Input: part model. Units: mm. Frame: model coordinates. A direction names the side the tool comes from. Coordinates: 2 decimals unless noted, no trailing zeros. Write each loop counter-clockwise with the first axis right and the second up, starting at its lowest first coordinate (ties: lowest second). Pieces come first, ordered by that corner, then holes. Notation, with made-up numbers: (-24.5, -28.75) - (-3.5, -28.75) arc R21 ccw to (-3.5, -22.75) - close; hole circle Ø6 at (66, 74). An arc over 180 degrees is marked (long way). Use CSV: the item, a comma, the result in double quotes.
```python
from build123d import *

# Parameters (mm, degrees)
BOSS_EXTRUDE1_DEPTH                             = 7.62
SKETCH11_W                                      = 17.78
SKETCH11_H                                      = 17.78
CUT_EXTRUDE1_DEPTH                              = 3.175
SKETCH12_W                                      = 3.81
SKETCH12_H                                      = 60.325
CUT_EXTRUDE2_DEPTH                              = 96.139869666
SKETCH14_W                                      = 7.62
SKETCH14_H                                      = 8.255
BOSS_EXTRUDE3_DEPTH                             = 3.175
SKETCH24_W                                      = 7.62
SKETCH24_H                                      = 6.35
BOSS_EXTRUDE4_DEPTH                             = 1.27
CSK_FOR_M3_FLAT_HEAD_MACHINE_SCREW2_D           = 3.4
CSK_FOR_M3_FLAT_HEAD_MACHINE_SCREW2_CSINK_D     = 6.3
CSK_FOR_M3_FLAT_HEAD_MACHINE_SCREW2_CSINK_ANGLE = 90
CSK_FOR_M3_FLAT_HEAD_MACHINE_SCREW3_D           = 3.4
CSK_FOR_M3_FLAT_HEAD_MACHINE_SCREW3_CSINK_D     = 6.3
CSK_FOR_M3_FLAT_HEAD_MACHINE_SCREW3_CSINK_ANGLE = 90
F_4_40_TAPPED_HOLE2_D                           = 2.2606
F_4_40_TAPPED_HOLE2_DEPTH                       = 8.8646
F_4_40_TAPPED_HOLE2_TIP                         = 0.679152758
SKETCH25_W                                      = 5.08
SKETCH25_H                                      = 93.98
CUT_EXTRUDE3_DEPTH                              = 96.139869666
FILLET1_R                                       = 3.302


with BuildPart() as part:
    # Sketch1 → Boss-Extrude1 (new body)
    with BuildSketch(Plane.XY):
        Polygon((0, -93.98), (0, -7.62), (-5.08, -7.62), (-5.08, 0), (12.7, 0), (12.7, -7.62), (7.62, -7.62), (7.62, -93.98), align=None)
    extrude(amount=BOSS_EXTRUDE1_DEPTH)

    # Sketch11 → Cut-Extrude1 (cut)
    with BuildSketch(Plane.XY.offset(7.62)):
        with Locations((3.81, -8.89)):
            Rectangle(SKETCH11_W, SKETCH11_H)
    extrude(amount=-CUT_EXTRUDE1_DEPTH, mode=Mode.SUBTRACT)

    # Sketch12 → Cut-Extrude2 (cut, through all)
    with BuildSketch(Plane(origin=(7.62, 0, 0), x_dir=(0, 0, -1), z_dir=(1, 0, 0))):
        with Locations((-1.905, -55.5625)):
            Rectangle(SKETCH12_W, SKETCH12_H)
    extrude(amount=-CUT_EXTRUDE2_DEPTH, mode=Mode.SUBTRACT)

    # Sketch14 → Boss-Extrude3 (add)
    with BuildSketch(Plane(origin=(7.62, 0, 0), x_dir=(0, 0, -1), z_dir=(1, 0, 0))):
        with Locations((-3.81, -89.8525)):
            Rectangle(SKETCH14_W, SKETCH14_H)
    boss_extrude3 = extrude(amount=BOSS_EXTRUDE3_DEPTH)

    # Mirror1: Boss-Extrude3 across plane
    add(boss_extrude3.mirror(Plane(origin=(3.81, 0, 0), x_dir=(0, 0, 1), z_dir=(1, 0, 0))))

    # Sketch24 → Boss-Extrude4 (add)
    with BuildSketch(Plane(origin=(0, 0, 3.81), x_dir=(-1, 0, 0), z_dir=(0, 0, -1))):
        with Locations((-3.81, -82.55)):
            Rectangle(SKETCH24_W, SKETCH24_H)
    extrude(amount=BOSS_EXTRUDE4_DEPTH)

    # CSK for M3 Flat Head Machine Screw2 (through all)
    with Locations(Plane.XY.offset(7.62)):
        with Locations((1.27, -89.535)):
            CounterSinkHole(CSK_FOR_M3_FLAT_HEAD_MACHINE_SCREW2_D / 2, CSK_FOR_M3_FLAT_HEAD_MACHINE_SCREW2_CSINK_D / 2, counter_sink_angle=CSK_FOR_M3_FLAT_HEAD_MACHINE_SCREW2_CSINK_ANGLE)

    # CSK for M3 Flat Head Machine Screw3 (through all)
    with Locations(Plane.XY.offset(4.445)):
        with Locations((-1.905, -3.81)):
            CounterSinkHole(CSK_FOR_M3_FLAT_HEAD_MACHINE_SCREW3_D / 2, CSK_FOR_M3_FLAT_HEAD_MACHINE_SCREW3_CSINK_D / 2, counter_sink_angle=CSK_FOR_M3_FLAT_HEAD_MACHINE_SCREW3_CSINK_ANGLE)

    # #4-40 Tapped Hole2
    with Locations(Plane(origin=(7.62, 0, 0), x_dir=(0, 0, -1), z_dir=(1, 0, 0))):
        with Locations((-5.08, -20.9677), (-5.08, -81.9277)):
            Hole(F_4_40_TAPPED_HOLE2_D / 2, depth=F_4_40_TAPPED_HOLE2_DEPTH)
            with Locations((0, 0, -(F_4_40_TAPPED_HOLE2_DEPTH + F_4_40_TAPPED_HOLE2_TIP / 2))):  # 118° drill point
                Cone(0, F_4_40_TAPPED_HOLE2_D / 2, F_4_40_TAPPED_HOLE2_TIP, mode=Mode.SUBTRACT)

    # Sketch25 → Cut-Extrude3 (cut, through all)
    with BuildSketch(Plane(origin=(0, 0, 0), x_dir=(-1, 0, 0), z_dir=(0, 0, -1))):
        with Locations((-10.16, -46.99)):
            Rectangle(SKETCH25_W, SKETCH25_H)
    extrude(amount=-CUT_EXTRUDE3_DEPTH, mode=Mode.SUBTRACT)

    # Fillet1
    # the kernel refuses this fillet: 3.302 mm, written as the material it adds along each edge
    with BuildSketch(Plane(origin=(7.62, -85.725, 2.54), x_dir=(0, 0, -1), z_dir=(-1, 0, 0))) as fillet1_piece_1:
        with BuildLine():
            CenterArc((3.302, -3.212874103), FILLET1_R, 103.342363797, 76.657636203)
            Line((0, -3.212874103), (-0.06604, -3.212874103))
            Line((-0.06604, -3.212874103), (-0.06604, 0))
            Line((-0.06604, 0), (0, 0.06604))
            ThreePointArc((0, 0.06604), (1.27, 0.06604), (2.52476, 0.064257482))
            Line((2.52476, 0.064257482), (2.54, 0))
        make_face()
    extrude(amount=7.62)
    with BuildSketch(Plane(origin=(0, -79.375, 3.81), x_dir=(0, 0, -1), z_dir=(1, 0, 0))) as fillet1_piece_2:
        with BuildLine():
            CenterArc((3.302, 2.602725495), FILLET1_R, 180, 52.020127555)
            Line((0, 2.602725495), (-0.06604, 2.602725495))
            Line((-0.06604, 2.602725495), (-0.06604, 0))
            Line((-0.06604, 0), (0, -0.06604))
            ThreePointArc((0, -0.06604), (0.635, -0.06604), (1.22936, -0.05205451))
            Line((1.22936, -0.05205451), (1.27, 0))
        make_face()
    extrude(amount=7.62)
    with BuildSketch(Plane(origin=(7.62, -25.4, 3.81), x_dir=(0, 0, -1), z_dir=(-1, 0, 0))) as fillet1_piece_3:
        with BuildLine():
            CenterArc((FILLET1_R, FILLET1_R), FILLET1_R, 180, 90)
            Line((0, FILLET1_R), (-FILLET1_R * 0.02, FILLET1_R))
            Line((-FILLET1_R * 0.02, FILLET1_R), (-FILLET1_R * 0.02, -FILLET1_R * 0.02))
            Line((-FILLET1_R * 0.02, -FILLET1_R * 0.02), (FILLET1_R, -FILLET1_R * 0.02))
            Line((FILLET1_R, -FILLET1_R * 0.02), (FILLET1_R, 0))
        make_face()
    extrude(amount=7.62)
    with BuildSketch(Plane(origin=(7.62, -17.78, 4.445), x_dir=(0, 0, 1), z_dir=(-1, 0, 0))) as fillet1_piece_4:
        with BuildLine():
            CenterArc((3.302, 3.299556788), FILLET1_R, 180, 87.795772496)
            Line((0, 3.299556788), (-0.06604, 3.299556788))
            Line((-0.06604, 3.299556788), (-0.06604, 0))
            Line((-0.06604, 0), (0, -0.06604))
            ThreePointArc((0, -0.06604), (1.5875, -0.06604), (3.17246, -0.065991136))
            Line((3.17246, -0.065991136), (3.175, 0))
        make_face()
    extrude(amount=7.62)


solid = part.part
```
(1) Cut plane B-B on x = 5.25. Return loops of the section in (y, z) (3 decimals).
Check values:
outline,"(-93.98, 0) - (-85.725, 0) arc R3.302 cw to (-82.512, 2.54) - (-79.375, 2.54) arc R3.302 cw to (-76.772, 3.81) - (-28.702, 3.81) arc R3.302 cw to (-25.4, 0.508) - (-25.4, 0) - (0, 0) - (0, 4.445) - (-14.48, 4.445) arc R3.302 cw to (-17.78, 7.62) - (-93.98, 7.62) - close; hole circle Ø2.261 at (-81.928, 5.08); hole circle Ø2.261 at (-20.968, 5.08)"
(2) Cut plane A-A on y = -3.81. Return loops of the section in (x, z) (3 decimals), and give its area (3 significant figures).
Check values:
outline,"(-5.08, 0) - (-3.605, 0) - (-3.605, 2.995) - (-5.055, 4.445) - (-5.08, 4.445) - close; (-0.205, 0) - (7.62, 0) - (7.62, 4.445) - (1.245, 4.445) - (-0.205, 2.995) - close"
area,"39.2 mm^2"
(3) Pin query (flat end, axial travel): pin 1 Ø3 at (y, z) = (-81.93, 5.08) entering from -X; pin 2 Ø1.4 at (y, z) = (-20.97, 5.08) entering from +X; pin 3 Ø5.5 at (x, y) = (-1.905, -3.81) entering from +Z (3 decimals); pin 4 Ø4 at (x, y) = (0, -5.5) entering from +Z (3 decimals). Return the tip coordinate at first contact, or that it passes through.
Check values:
pin 1,"x = 0"
pin 2,"through"
pin 3,"z = 4.045"
pin 4,"z = 4.445"
(4) Draft query along Y for faces 1 (the flat face through (4, -81, 2.54)), 2 (the flat face through (2, -93.98, 4)), 3 (the cylindrical face through (3.757, -19.847, 4.933)), 4 (the flat face through (3, -10, 0)). Return one class per face: pulls with the +Y half, pulls with the -Y half, needs draft (parallel to the pull), parting line crosses it, or undercut.
Check values:
face 1,"undercut"
face 2,"pulls with the -Y half"
face 3,"undercut"
face 4,"needs draft"
(5) Ray query, probe 1 along Y at (x, z) = (-1.75, 1.75) (3 decimals); probe 2 along Y at (x, z) = (2, 3.5); probe 3 along Y at (x, z) = (2.5, 4.75). Return the intervals inside material, ascending. Write a range as from..to.
Check values:
probe 1,"-93.98..-85.725, -7.62..-5.503, -2.117..0"
probe 2,"-93.98..-91.07, -88..-78.17, -27.31..0"
probe 3,"-93.98..-90.71, -88.36..-83.01, -80.85..-22.05, -19.89..-15.87"
(6) Cut plane C-C on y = -61.5. Return loops of the section in (x, z), and give its area (3 significant figures).
Check values:
outline,"(0, 3.81) - (7.62, 3.81) - (7.62, 7.62) - (0, 7.62) - close"
area,"29.0 mm^2"
(7) Reachability of faces 5 (the flat face through (3, -7, 4.445)), 6 (the flat face through (4, -53, 3.81)), 7 (the flat face through (-3.175, -90, 4)) from +Z, -Z, +X, -X, +Y, -Y: full face, straight path, thin tool, end or side. Return the list, or none.
Check values:
face 5,"+Z, +X, -X, +Y"
face 6,"-Z, +X, -X"
face 7,"+Z, -Z, -X, -Y"
